Verification items for the finished model (mm, model axes). A direction names the side the tool comes from. Give positions to 0.01 mm unless a question says otherwise; leave off trailing zeros. Order: outer loops, then holes, each group sorted by start corner. A loop starts at its lowest first (then second) coordinate and runs counter-clockwise, first axis right, second up. Notation, with made-up numbers: (42.25, 53) -> (56.25, 53) arc R11 cw to (56.25, 62) -> close; hole circle Ø1 at (78, 79). An arc over 180 degrees is marked (long way). Return JSON: item names as keys, results as strings. Group by question number.
(1) Depth check by flat-ended pin: pin 1 Ø8.5 at (x, z) = (336.55, 12.7) entering from -Y (3 decimals); pin 2 Ø1 at (x, z) = (-8, -20) entering from +Y. Enter the tip coordinate at first touch or a pass-through.
(2) Tool access check on faces 1 (the face through (231, 3.175, -12)), 2 (the face through (296.06, 0.04, -0.6)), 3 (the face through (0, 0, 0)). Record the directions out of +Z, -Z, +X, -X, +Y, -Y that give a thin tool (end or side, any length) a straight path to the whole face; none if there is none.
(3) Thickness scan on line 1 along Z through (x, y) = (-349.25, 1) (3 decimals); line 2 along Z through (x, y) = (19.05, -0.7) (3 decimals); line 3 along X through (y, z) = (0.25, -24.5) (3 decimals). Record the ranges inside material, lowest first.
(4) Release check for a two-part mould opening along X. For faces 4 (the face through (-296.06, 0.04, -0.6)), 5 (the face through (-190, 3.175, 19)) record: pulls with the +X half, pulls with the -X half, needs draft (parallel to the pull), parting line crosses it, or undercut.
(5) Cross-section at A-A on x = 210. Enter the section's corners in (y, z) (3 decimals), then the cut area to 3 significant figures.
(6) Cross-section at B-B on y = 1.5. State how many separate pieces and enclosed holes the cut face has, then the cut area to 3 significant figures.
from build123d import *

# Parameters (mm, degrees)
SKETCH2_W                   = 57.15
SKETCH2_H                   = 6.35
BOSS_EXTRUDE2_DEPTH         = 355.6
F_1_4_0_25_DIAMETER_HOLE1_D = 6.35
CUT_EXTRUDE1_REACH          = 358.803
FILLET1_R                   = 3.175
FILLET1_OF_MIRROR1_R        = 3.175
SKETCH7_W                   = 57.15
SKETCH7_H                   = 57.15
CUT_EXTRUDE2_DEPTH          = 3.175
F_1_4_0_25_DIAMETER_HOLE2_D = 6.35


with BuildPart() as part:
    # Sketch2 → Boss-Extrude2 (new, symmetric)
    with BuildSketch(Plane(origin=(0, 0, 0), x_dir=(0, 0, -1), z_dir=(1, 0, 0))):
        Rectangle(SKETCH2_W, SKETCH2_H)
    extrude(amount=BOSS_EXTRUDE2_DEPTH, both=True)

    # 1/4 (0.25) Diameter Hole1 (through all)
    with Locations(Plane(origin=(0, 3.175, 0), x_dir=(1, 0, 0), z_dir=(0, 1, 0))):
        with Locations((-349.25, -12.7), (-349.25, 12.7), (-336.55, 12.7), (-336.55, -12.7)):
            f_1_4_0_25_diameter_hole1 = Hole(F_1_4_0_25_DIAMETER_HOLE1_D / 2)

    # Sketch6 → Cut-Extrude1 (cut, up to next)
    with BuildSketch(Plane(origin=(0, 3.175, 0), x_dir=(1, 0, 0), z_dir=(0, 1, 0)), mode=Mode.PRIVATE) as cut_extrude1_sk1:
        Polygon((-323.85, 22.225), (-323.85, -22.225), (-266.721810637, -22.225), align=None)
    cut_extrude1_tool1 = extrude(cut_extrude1_sk1.sketch, amount=-CUT_EXTRUDE1_REACH, mode=Mode.PRIVATE) & part.part
    # Sketch6 → Cut-Extrude1 (cut, up to next)
    with BuildSketch(Plane(origin=(0, 3.175, 0), x_dir=(1, 0, 0), z_dir=(0, 1, 0)), mode=Mode.PRIVATE) as cut_extrude1_sk2:
        Polygon((-313.509439363, 22.225), (-256.38125, -22.225), (-256.38125, 22.225), align=None)
    cut_extrude1_tool2 = extrude(cut_extrude1_sk2.sketch, amount=-CUT_EXTRUDE1_REACH, mode=Mode.PRIVATE) & part.part
    # Sketch6 → Cut-Extrude1 (cut, up to next)
    with BuildSketch(Plane(origin=(0, 3.175, 0), x_dir=(1, 0, 0), z_dir=(0, 1, 0)), mode=Mode.PRIVATE) as cut_extrude1_sk3:
        Polygon((-250.03125, 22.225), (-250.03125, -22.225), (-192.903060637, -22.225), align=None)
    cut_extrude1_tool3 = extrude(cut_extrude1_sk3.sketch, amount=-CUT_EXTRUDE1_REACH, mode=Mode.PRIVATE) & part.part
    # Sketch6 → Cut-Extrude1 (cut, up to next)
    with BuildSketch(Plane(origin=(0, 3.175, 0), x_dir=(1, 0, 0), z_dir=(0, 1, 0)), mode=Mode.PRIVATE) as cut_extrude1_sk4:
        Polygon((-239.690689363, 22.225), (-182.5625, -22.225), (-182.5625, 22.225), align=None)
    cut_extrude1_tool4 = extrude(cut_extrude1_sk4.sketch, amount=-CUT_EXTRUDE1_REACH, mode=Mode.PRIVATE) & part.part
    # Sketch6 → Cut-Extrude1 (cut, up to next)
    with BuildSketch(Plane(origin=(0, 3.175, 0), x_dir=(1, 0, 0), z_dir=(0, 1, 0)), mode=Mode.PRIVATE) as cut_extrude1_sk5:
        Polygon((-176.2125, 22.225), (-176.2125, -22.225), (-119.084310637, -22.225), align=None)
    cut_extrude1_tool5 = extrude(cut_extrude1_sk5.sketch, amount=-CUT_EXTRUDE1_REACH, mode=Mode.PRIVATE) & part.part
    # Sketch6 → Cut-Extrude1 (cut, up to next)
    with BuildSketch(Plane(origin=(0, 3.175, 0), x_dir=(1, 0, 0), z_dir=(0, 1, 0)), mode=Mode.PRIVATE) as cut_extrude1_sk6:
        Polygon((-165.871939363, 22.225), (-108.74375, -22.225), (-108.74375, 22.225), align=None)
    cut_extrude1_tool6 = extrude(cut_extrude1_sk6.sketch, amount=-CUT_EXTRUDE1_REACH, mode=Mode.PRIVATE) & part.part
    # Sketch6 → Cut-Extrude1 (cut, up to next)
    with BuildSketch(Plane(origin=(0, 3.175, 0), x_dir=(1, 0, 0), z_dir=(0, 1, 0)), mode=Mode.PRIVATE) as cut_extrude1_sk7:
        Polygon((-102.39375, 22.225), (-102.39375, -22.225), (-45.265560637, -22.225), align=None)
    cut_extrude1_tool7 = extrude(cut_extrude1_sk7.sketch, amount=-CUT_EXTRUDE1_REACH, mode=Mode.PRIVATE) & part.part
    # Sketch6 → Cut-Extrude1 (cut, up to next)
    with BuildSketch(Plane(origin=(0, 3.175, 0), x_dir=(1, 0, 0), z_dir=(0, 1, 0)), mode=Mode.PRIVATE) as cut_extrude1_sk8:
        Polygon((-92.053189363, 22.225), (-34.925, -22.225), (-34.925, 22.225), align=None)
    cut_extrude1_tool8 = extrude(cut_extrude1_sk8.sketch, amount=-CUT_EXTRUDE1_REACH, mode=Mode.PRIVATE) & part.part
    cut_extrude1_1 = cut_extrude1_tool1.solids().sort_by_distance((-304.80727, 3.175, 7.408333))[0]
    add(cut_extrude1_1, mode=Mode.SUBTRACT)
    cut_extrude1_2 = cut_extrude1_tool2.solids().sort_by_distance((-275.42398, 3.175, -7.408333))[0]
    add(cut_extrude1_2, mode=Mode.SUBTRACT)
    cut_extrude1_3 = cut_extrude1_tool3.solids().sort_by_distance((-230.98852, 3.175, 7.408333))[0]
    add(cut_extrude1_3, mode=Mode.SUBTRACT)
    cut_extrude1_4 = cut_extrude1_tool4.solids().sort_by_distance((-201.60523, 3.175, -7.408333))[0]
    add(cut_extrude1_4, mode=Mode.SUBTRACT)
    cut_extrude1_5 = cut_extrude1_tool5.solids().sort_by_distance((-157.16977, 3.175, 7.408333))[0]
    add(cut_extrude1_5, mode=Mode.SUBTRACT)
    cut_extrude1_6 = cut_extrude1_tool6.solids().sort_by_distance((-127.78648, 3.175, -7.408333))[0]
    add(cut_extrude1_6, mode=Mode.SUBTRACT)
    cut_extrude1_7 = cut_extrude1_tool7.solids().sort_by_distance((-83.35102, 3.175, 7.408333))[0]
    add(cut_extrude1_7, mode=Mode.SUBTRACT)
    cut_extrude1_8 = cut_extrude1_tool8.solids().sort_by_distance((-53.96773, 3.175, -7.408333))[0]
    add(cut_extrude1_8, mode=Mode.SUBTRACT)
    cut_extrude1 = cut_extrude1_1 + cut_extrude1_2 + cut_extrude1_3 + cut_extrude1_4 + cut_extrude1_5 + cut_extrude1_6 + cut_extrude1_7 + cut_extrude1_8  # Cut-Extrude1 as one shape, for the pattern or mirror that repeats it

    # Fillet1
    fillet1_edges = [part.edges().sort_by_distance(p)[0] for p in [
        (-92.053189363, 0, -22.225),
        (-34.925, 0, -22.225),
        (-34.925, 0, 22.225),
        (-323.85, 0, -22.225),
        (-266.721810637, 0, 22.225),
        (-323.85, 0, 22.225),
        (-313.509439363, 0, -22.225),
        (-256.38125, 0, -22.225),
        (-256.38125, 0, 22.225),
        (-250.03125, 0, -22.225),
        (-192.903060637, 0, 22.225),
        (-250.03125, 0, 22.225),
        (-239.690689363, 0, -22.225),
        (-182.5625, 0, -22.225),
        (-182.5625, 0, 22.225),
        (-176.2125, 0, -22.225),
        (-119.084310637, 0, 22.225),
        (-176.2125, 0, 22.225),
        (-165.871939363, 0, -22.225),
        (-108.74375, 0, -22.225),
        (-108.74375, 0, 22.225),
        (-102.39375, 0, -22.225),
        (-45.265560637, 0, 22.225),
        (-102.39375, 0, 22.225),
    ]]
    fillet(fillet1_edges, radius=FILLET1_R)

    # Mirror1: 1/4 (0.25) Diameter Hole1, Cut-Extrude1 across plane
    add(f_1_4_0_25_diameter_hole1.mirror(Plane(origin=(0, 0, 0), x_dir=(0, 0, 1), z_dir=(1, 0, 0))), mode=Mode.SUBTRACT)
    add(cut_extrude1.mirror(Plane(origin=(0, 0, 0), x_dir=(0, 0, 1), z_dir=(1, 0, 0))), mode=Mode.SUBTRACT)

    # Fillet1 of Mirror1
    fillet1_of_mirror1_edges = [part.edges().sort_by_distance(p)[0] for p in [
        (92.053189363, 0, -22.225),
        (34.925, 0, -22.225),
        (34.925, 0, 22.225),
        (323.85, 0, -22.225),
        (266.721810637, 0, 22.225),
        (323.85, 0, 22.225),
        (313.509439363, 0, -22.225),
        (256.38125, 0, -22.225),
        (256.38125, 0, 22.225),
        (250.03125, 0, -22.225),
        (192.903060637, 0, 22.225),
        (250.03125, 0, 22.225),
        (239.690689363, 0, -22.225),
        (182.5625, 0, -22.225),
        (182.5625, 0, 22.225),
        (176.2125, 0, -22.225),
        (119.084310637, 0, 22.225),
        (176.2125, 0, 22.225),
        (165.871939363, 0, -22.225),
        (108.74375, 0, -22.225),
        (108.74375, 0, 22.225),
        (102.39375, 0, -22.225),
        (45.265560637, 0, 22.225),
        (102.39375, 0, 22.225),
    ]]
    fillet(fillet1_of_mirror1_edges, radius=FILLET1_OF_MIRROR1_R)

    # Sketch7 → Cut-Extrude2 (cut)
    with BuildSketch(Plane(origin=(0, 3.175, 0), x_dir=(1, 0, 0), z_dir=(0, 1, 0))):
        Rectangle(SKETCH7_W, SKETCH7_H)
    extrude(amount=-CUT_EXTRUDE2_DEPTH, mode=Mode.SUBTRACT)

    # 1/4 (0.25) Diameter Hole2 (through all)
    with Locations(Plane(origin=(0, 0, 0), x_dir=(1, 0, 0), z_dir=(0, 1, 0))):
        with Locations((19.05, -19.05), (-19.05, 19.05), (-19.05, -19.05), (19.05, 19.05)):
            Hole(F_1_4_0_25_DIAMETER_HOLE2_D / 2)


solid = part.part
Verdict:
{
 "1": {"pin 1": "y = -3.175", "pin 2": "y = 0"},
 "2": {"face 1": "+Z, -Z, +X, -X, +Y", "face 2": "+Y, -Y", "face 3": "+Z, -Z, +Y"},
 "3": {"line 1": "-28.575 to -15.875, -9.525 to 9.525, 15.875 to 28.575", "line 2": "-28.575 to -22.225, -15.875 to 15.875, 22.225 to 28.575", "line 3": "-355.6 to -28.575, 28.575 to 355.6"},
 "4": {"face 4": "undercut", "face 5": "needs draft"},
 "5": {"outline": "(-3.175, -28.575) -> (3.175, -28.575) -> (3.175, -22.225) -> (-3.175, -22.225) -> close; (-3.175, 0.877) -> (3.175, 0.877) -> (3.175, 8.922) -> (-3.175, 8.922) -> close; (-3.175, 22.225) -> (3.175, 22.225) -> (3.175, 28.575) -> (-3.175, 28.575) -> close", "area": "132 mm²"},
 "6": {"separate pieces": "2", "enclosed holes": "24", "area": "17,300 mm²"}
}
